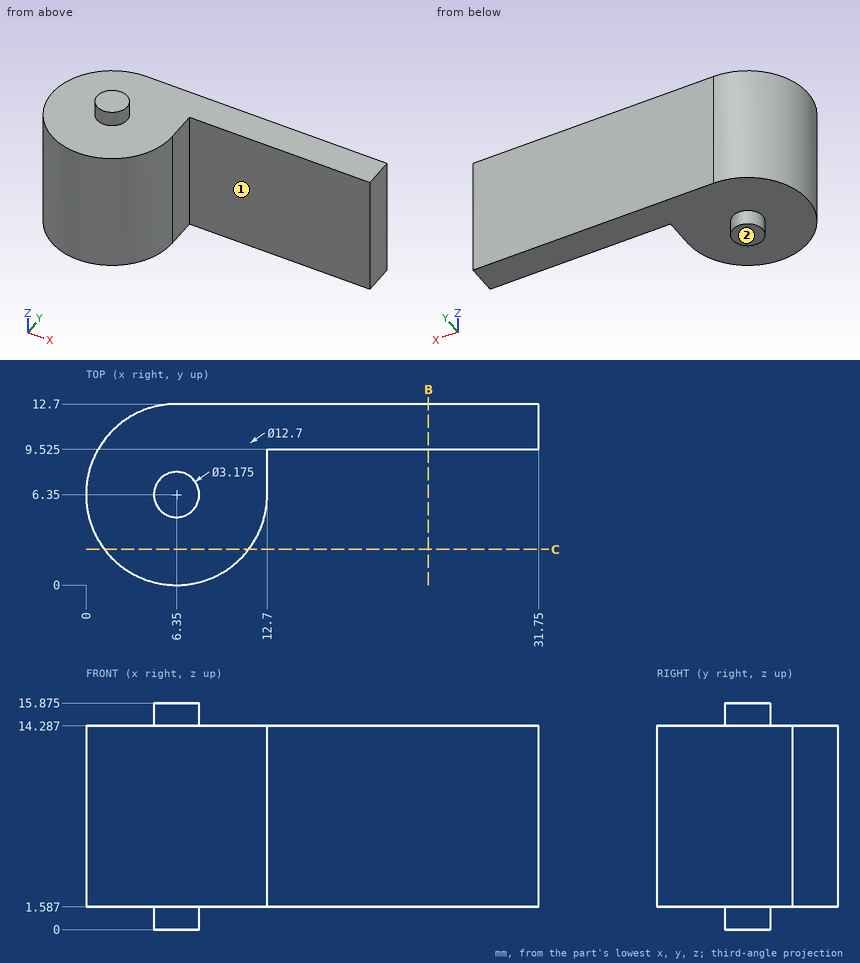
Source: three-view drawing plus pictorial views. Frame: mm from the lowest corner of the part. A direction names the side the tool comes from. Round coordinates to 2 decimals unless told otherwise and drop trailing zeros. Write each loop counter-clockwise with the first axis right and the second up, starting at its lowest first coordinate (ties: lowest second). Pieces come first, ordered by that corner, then holes. Notation, with made-up numbers: M 13,-9.75 L 25,-9.75 A30 ccw 25,26.25 Z; hole C 30,3.5 d11. An arc over 180 degrees is marked long. One line per item, written item: value. Start each with the question number.
Item 1: Set-up query: the marked faces 1 and 2. Return all of +Z, -Z, +X, -X, +Y, -Y with unobstructed straight access to the full face (end or side cutting, diameter ignored); none if empty.
Item 2: Section query B-B (x = 24). Return the cut outline in (y, z) (1 decimal).
Item 3: Ray query, L1, parallel to Z at x = 9.5, y = 4; L2, parallel to Y at x = 24, z = 11.5 (1 decimal); L3, parallel to X at y = 6.5, z = 11.25. Return the intervals inside material, ascending. Write a range as from..to.
Item 4: Pin query (flat end, axial travel): pin 1 (3.5 mm diameter, centred on y = 8.5, z = 5.5, fed in from +X); pin 2 (1.5 mm diameter, centred on y = 2.5, z = 7, fed in from +X); pin 3 (1 mm diameter, centred on y = 8.5, z = 5.5, fed in from -X); pin 4 (1 mm diameter, centred on y = 4, z = 11.5, fed in from +X) (1 decimal). Return the tip coordinate at first contact, or that it passes through.
Item 5: Section query C-C (y = 2.5). Return the cut outline in (x, z), plus the area to 3 significant figures.
Result set:
1. face 1: +Z, -Z, +X, -Y
1. face 2: -Z, +X, -X, +Y, -Y
2. outline: M 9.5,1.6 L 12.7,1.6 L 12.7,14.3 L 9.5,14.3 Z
3. L1: z = 1.59..14.29
3. L2: y = 9.5..12.7
3. L3: x = 0..12.7
4. pin 1: stops at x = 31.75
4. pin 2: stops at x = 11.89
4. pin 3: stops at x = 0.22
4. pin 4: stops at x = 12.4
5. outline: M 1.3,1.59 L 11.4,1.59 L 11.4,14.29 L 1.3,14.29 Z
5. area: 128 mm²
